Here's how the part is built. I have some questions about the finished solid (model axes, mm). Round coordinates to 2 decimals unless told otherwise and drop trailing zeros. Write each loop counter-clockwise with the first axis right and the second up, starting at its lowest first coordinate (ties: lowest second). Pieces come first, ordered by that corner, then holes. Notation, with made-up numbers: (32, -34) -> (67, -34) arc R32 cw to (67, 2) -> close; hole circle Ø5 at (70, 83.5). An arc over 180 degrees is marked (long way). Put each result on its own line as item: value. Start each with the question number.
1. I need wall thicknesses on probe 1 along Z at (x, y) = (0, -1.85); probe 2 along Z at (x, y) = (1, -0.9); probe 3 along X at (y, z) = (-0.05, 21.8). Which ranges of each line are inside material? Lowest first, please. Write a range as from..to.
2. For pin 1 (1.7 mm diameter, centred on x = 0, z = 21.8, fed in from -Y); pin 2 (1.5 mm diameter, centred on y = 1.5, z = 118, fed in from -X), each with a flat end and sliding along its axis, tell me the tip position at first contact or that it passes through.
3. We'd pull the mould along X, two halves only. Please class faces 1 (the face through (-1.45, -0.47, 153.24)), 2 (the face through (0, -3, 79)), 3 (the face through (-1.45, -0.47, 21.74)), 4 (the face through (0, 0, 0)): +X half, -X half, draft (parallel to the pull), parting line (faces both ways), or undercut.
4. Suppose I cut it at C-C (z = 21.8). Please give me the cut outline in (x, y).
5. Suppose I cut it at B-B (y = 0). Please give me the cut outline in (x, z), then the cut area to 3 significant figures.
6. Suppose I cut it at A-A (x = 0). Please give me the cut outline in (y, z), then the cut area to 3 significant figures.
7. Suppose I cut it at D-D (z = 71). Please give me the cut outline in (x, y), then the cut area to 3 significant figures.
Autodesk Inventor part; units mm, degrees
ref_plane "YZ Plane" through (0, 0, 0) normal (1, 0, 0) x (0, 1, 0)
ref_plane "XZ Plane" through (0, 0, 0) normal (0, 1, 0) x (-1, 0, 0)
ref_plane "XY Plane" through (0, 0, 0) normal (0, 0, 1) x (1, 0, 0)
sketch "Sketch1" plane through (0, 0, 0) normal (0, 0, 1) x (1, 0, 0)
  circle A0 centre (0, 0) radius 3 construction
  line L0 (-2.2361, 2) -> (2.2361, 2)
  arc A1 (-2.2361, 2) -> (2.2361, 2) centre (0, 0) ccw
  dimension "d0" = 6
  dimension "d1" = 2
extrude "Extrusion1" add sketch "Sketch1" along normal blind 160
sketch "Sketch2" plane through (-2.2361, 2, 0) normal (0, 1, 0) x (1, 0, 0)
  circle A0 centre (2.2361, -157.9) radius 1.45
  line L0 (4.4721, -160) -> (0, -160)
  circle A1 centre (2.2361, -21.8) radius 1.45
  line L1 (0, 0) -> (4.4721, 0)
  circle A2 centre (2.2361, -26.4) radius 1.45
  circle A3 centre (2.2361, -153.3) radius 1.45
  point P0 (2.2361, 0)
  point P1 (2.2361, -160)
  point P2 (2.2361, 0)
  dimension "d4" = 2.9
  dimension "d5" = 2.1
  dimension "d8" = 2.9
  dimension "d9" = 21.8
  dimension "d10" = 2.9
  dimension "d11" = 4.6
  dimension "d12" = 2.9
  dimension "d13" = 4.6
extrude "Extrusion2" cut sketch "Sketch2" against normal through all
thread "Thread1"
thread "Thread2"
thread "Thread3"
thread "Thread4"
properties part number "6mm x 160mm D Shaft" material "Stainless Steel"
Verdict:
1. probe 1: z = 0..20.35, 23.25..24.95, 27.85..151.85, 154.75..156.45, 159.35..160
1. probe 2: z = 0..20.75, 22.85..25.35, 27.45..152.25, 154.35..156.85, 158.95..160
1. probe 3: x = -3..-1.45, 1.45..3
2. pin 1: passes through
2. pin 2: stops at x = -2.9
3. face 1: undercut
3. face 2: parting line
3. face 3: undercut
3. face 4: draft
4. outline: (-2.24, 2) arc R3 ccw to (-1.45, -2.63) -> (-1.45, 2) -> close; (1.45, -2.63) arc R3 ccw to (2.24, 2) -> (1.45, 2) -> close
5. outline: (-3, 0) -> (3, 0) -> (3, 160) -> (-3, 160) -> close; hole circle Ø2.9 at (0, 21.8); hole circle Ø2.9 at (0, 26.4); hole circle Ø2.9 at (0, 153.3); hole circle Ø2.9 at (0, 157.9)
5. area: 934 mm^2
6. outline: (-3, 0) -> (2, 0) -> (2, 20.35) -> (-3, 20.35) -> close; (-3, 23.25) -> (2, 23.25) -> (2, 24.95) -> (-3, 24.95) -> close; (-3, 27.85) -> (2, 27.85) -> (2, 151.85) -> (-3, 151.85) -> close; (-3, 154.75) -> (2, 154.75) -> (2, 156.45) -> (-3, 156.45) -> close; (-3, 159.35) -> (2, 159.35) -> (2, 160) -> (-3, 160) -> close
6. area: 742 mm^2
7. outline: (-2.24, 2) arc R3 ccw (long way) to (2.24, 2) -> close
7. area: 25.2 mm^2
